Geometry: final body of the model. Coordinates: model frame, mm. A direction names the side the tool comes from. Give positions to 0.01 mm unless a question says otherwise; leave off trailing zeros. Write each loop counter-clockwise with the first axis right and the second up, starting at its lowest first coordinate (ties: lowest second). Pieces come first, ordered by that corner, then holes. Notation, with made-up numbers: (-11.5, -21.5) -> (20.5, -21.5) arc R10 cw to (20.5, -8.5) -> close; hole circle Ø7 at (57, -4.75). An arc over 180 degrees is marked (long way). Answer as a JSON object with one key per item and string values. Group by question number.
(1) Draft query along X for faces 5 (the face through (-16.32, 38, 24)), 6 (the face through (-79.82, 38, 22)), 7 (the face through (-0.72, 18.96, 5.4)). Return one class per face: +X half, -X half, draft (parallel to the pull), parting line (faces both ways), or undercut.
(2) Section query C-C on y = 30.5. Output: boundary loops of the cut face in (x, z), plus the area to 3 significant figures.
(3) Section query B-B on x = -24.5. Output: boundary loops of the cut face in (y, z).
(4) Set-up query: faces 1 (the face through (-61, 38, 30.617)), 2 (the face through (-3, 0, 22)), 3 (the face through (-1, 38, 10.649)), 4 (the face through (39, 38, 38.1)). Return all of +Z, -Z, +X, -X, +Y, -Y with unobstructed straight access to the full face (end or side cutting, diameter ignored); none if empty.
(5) Section query A-A on z = 27. Output: boundary loops of the cut face in (x, y).
(6) Material intervals for probe 1 along X at (y, z) = (59.5, 36.5); probe 2 along X at (y, z) = (27, 27); probe 3 along Z at (x, y) = (-60, 27.5), sorted ascending.
(7) Contact query for flat-ended pins moving along their axis: pin 1 Ø4 at (x, y) = (-20, 31) entering from -Z; pin 2 Ø6 at (x, y) = (-37, 54) entering from +Z; pin 3 Ø23 at (x, y) = (26, 46) entering from +Z. Output: stop coordinate, or through.
(8) Section query D-D on x = 42. Output: boundary loops of the cut face in (y, z), plus the area to 3 significant figures.
from build123d import *

# Parameters (mm, degrees)
F1_DEPTH = 76.2
F3_DEPTH = 156.01986


with BuildPart() as f1:
    # F0 (on Front) → F1 (new body)
    with BuildSketch(Plane.XZ):
        Polygon((-76.2, 0), (0, 0), (76.2, 0), (76.2, 38.1), (0, 38.1), (-3.61986, 43.317194), (-29.01986, 43.317194), (-29.01986, 30.617194), (-16.31986, 30.617194), (-16.31986, 17.917194), (-67.11986, 17.917194), (-67.11986, 30.617194), (-54.41986, 30.617194), (-54.41986, 43.317194), (-79.81986, 43.317194), (-79.81986, 0), align=None)
    extrude(amount=-F1_DEPTH)

    # F2 (on face) → F3 (cut, through all)
    with BuildSketch(Plane.YZ.offset(76.2)):
        Polygon((63.5, 10.648813), (12.7, 10.648813), (25.4, 0), (50.8, 0), align=None)
    extrude(amount=-F3_DEPTH, mode=Mode.SUBTRACT)


solid = f1.part
Answer list:
{
 "1": {"face 5": "undercut", "face 6": "-X half", "face 7": "draft"},
 "2": {"outline": "(-79.82, 10.65) -> (76.2, 10.65) -> (76.2, 38.1) -> (0, 38.1) -> (-3.62, 43.32) -> (-29.02, 43.32) -> (-29.02, 30.62) -> (-16.32, 30.62) -> (-16.32, 17.92) -> (-67.12, 17.92) -> (-67.12, 30.62) -> (-54.42, 30.62) -> (-54.42, 43.32) -> (-79.82, 43.32) -> close", "area": "3,720 mm2"},
 "3": {"outline": "(0, 0) -> (25.4, 0) -> (12.7, 10.65) -> (63.5, 10.65) -> (50.8, 0) -> (76.2, 0) -> (76.2, 17.92) -> (0, 17.92) -> close; (0, 30.62) -> (76.2, 30.62) -> (76.2, 43.32) -> (0, 43.32) -> close"},
 "4": {"face 1": "+Y, -Y", "face 2": "+Z, -Z, +X, -X, -Y", "face 3": "+X, -X", "face 4": "+Z, +X, +Y, -Y"},
 "5": {"outline": "(-79.82, 0) -> (-67.12, 0) -> (-67.12, 76.2) -> (-79.82, 76.2) -> close; (-16.32, 0) -> (76.2, 0) -> (76.2, 76.2) -> (-16.32, 76.2) -> close"},
 "6": {"probe 1": "-79.82 to -54.42, -29.02 to 76.2", "probe 2": "-79.82 to -67.12, -16.32 to 76.2", "probe 3": "10.65 to 17.92, 30.62 to 43.32"},
 "7": {"pin 1": "z = 10.65", "pin 2": "z = 17.92", "pin 3": "z = 38.1"},
 "8": {"outline": "(0, 0) -> (25.4, 0) -> (12.7, 10.65) -> (63.5, 10.65) -> (50.8, 0) -> (76.2, 0) -> (76.2, 38.1) -> (0, 38.1) -> close", "area": "2,500 mm2"}
}
